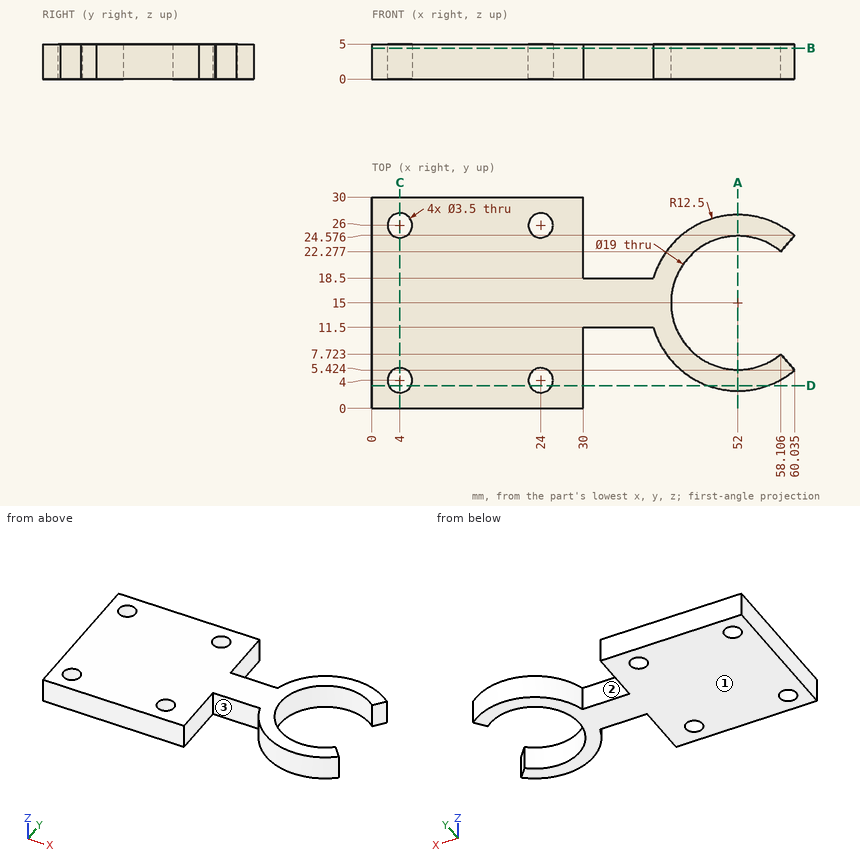
Design review of the part shown in the three views and the two pictorial views. Dimensions are in mm from the part's minimum x, y and z. Coordinates: 2 decimals unless noted, no trailing zeros. Write each loop counter-clockwise with the first axis right and the second up, starting at its lowest first coordinate (ties: lowest second). Pieces come first, ordered by that corner, then holes.
(1) For pin 1 Ø4 at (x, y) = (4, 26) entering from -Z; pin 2 Ø3 at (x, y) = (24, 26) entering from +Z; pin 3 Ø2 at (x, z) = (32, 4) entering from +Y; pin 4 Ø2.5 at (x, z) = (33.5, 3) entering from -Y, all flat-tipped, find the tip position at first contact; note any pin that passes through.
(2) The part is to be moulded in two halves that separate along X. For the marked faces 1, 2 and 3, say which applies: +X half, -X half, draft (parallel to the pull), parting line (faces both ways), or undercut.
(3) Add section A-A on x = 52. Give the boundary of the cut face in (y, z).
(4) Wall thickness on probe 1 along Y at (x, z) = (4, 2); probe 2 along Y at (x, z) = (52, 2.5); probe 3 along X at (y, z) = (2, 3.8): over which ranges is each line inside the solid? List them lowest first.
(5) Add section B-B on z = 4.4. Count the separate pieces of the cut face and the enclosed holes in it, then the cut area to 3 significant figures.
(6) Add section C-C on x = 4. Give the boundary of the cut face in (y, z).
(7) Add section D-D on y = 3.25. Give the boundary of the cut face in (x, z) (1 decimal).
Answer sheet:
1. pin 1: stops at z = 0
1. pin 2: passes through
1. pin 3: stops at y = 18.5
1. pin 4: stops at y = 11.5
2. face 1: draft
2. face 2: undercut
2. face 3: undercut
3. outline: (2.5, 0) - (5.5, 0) - (5.5, 5) - (2.5, 5) - close; (24.5, 0) - (27.5, 0) - (27.5, 5) - (24.5, 5) - close
4. probe 1: y = 0 to 2.25, 5.75 to 24.25, 27.75 to 30
4. probe 2: y = 2.5 to 5.5, 24.5 to 27.5
4. probe 3: x = 0 to 30
5. separate pieces: 1
5. enclosed holes: 4
5. area: 1,080 mm2
6. outline: (0, 0) - (2.25, 0) - (2.25, 5) - (0, 5) - close; (5.75, 0) - (24.25, 0) - (24.25, 5) - (5.75, 5) - close; (27.75, 0) - (30, 0) - (30, 5) - (27.75, 5) - close
7. outline: (0, 0) - (2.4, 0) - (2.4, 5) - (0, 5) - close; (5.6, 0) - (22.4, 0) - (22.4, 5) - (5.6, 5) - close; (25.6, 0) - (30, 0) - (30, 5) - (25.6, 5) - close; (47.7, 0) - (56.3, 0) - (56.3, 5) - (47.7, 5) - close
